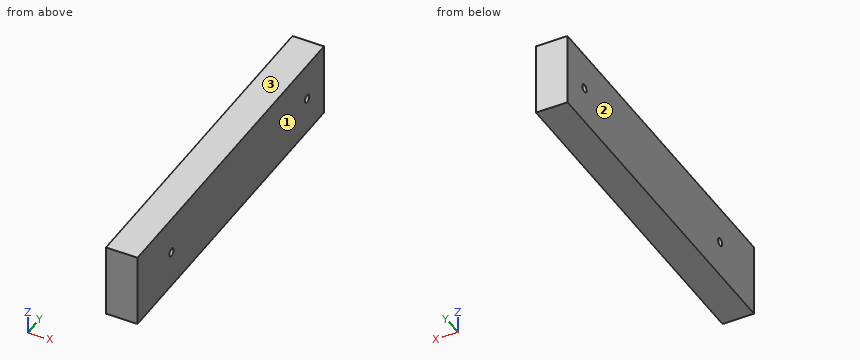
```python
from build123d import *

# Parameters (mm, degrees)
SKETCH1_W           = 38.1
SKETCH1_H           = 88.9
BOSS_EXTRUDE1_DEPTH = 419.1
SKETCH2_OUTSIDE_W   = 176.924
SKETCH2_OUTSIDE_H   = 507.124
SKETCH2_OUTSIDE_W_2 = 88.9
SKETCH2_OUTSIDE_H_2 = 419.1
SKETCH2_OUTSIDE_R   = 4.7625
CUT_EXTRUDE1_DEPTH  = 38.1


with BuildPart() as part:
    # Sketch1 → Boss-Extrude1 (new body)
    with BuildSketch(Plane(origin=(0, 0, 0), x_dir=(1, 0, 0), z_dir=(0, 1, 0))):
        with Locations((19.05, 44.45)):
            Rectangle(SKETCH1_W, SKETCH1_H)
    extrude(amount=BOSS_EXTRUDE1_DEPTH)

    # Sketch2 outside → Cut-Extrude1 (cut)
    # profile 1 of 3: a face of its own
    with BuildSketch(Plane.ZY):
        with Locations((-44.45, 209.55)):
            Rectangle(SKETCH2_OUTSIDE_W, SKETCH2_OUTSIDE_H)
        with Locations((-44.45, 209.55)):
            Rectangle(SKETCH2_OUTSIDE_W_2, SKETCH2_OUTSIDE_H_2, mode=Mode.SUBTRACT)
    # profile 2 of 3: a face of its own
    with BuildSketch(Plane.ZY):
        with Locations((-44.45, 381)):
            Circle(SKETCH2_OUTSIDE_R)
    # profile 3 of 3: a face of its own
    with BuildSketch(Plane.ZY):
        with Locations((-44.45, 76.2)):
            Circle(SKETCH2_OUTSIDE_R)
    extrude(amount=-CUT_EXTRUDE1_DEPTH, mode=Mode.SUBTRACT)


solid = part.part
```
Could you check a few things on this model? Use its own coordinates, in mm. Face numbers are marked on the shaded views. Round coordinates to 2 decimals unless told otherwise and drop trailing zeros. Loops run counter-clockwise (first coordinate to the right, second up) from the corner with the lowest first, then second, coordinate; pieces in that order, holes last. Notation, with made-up numbers: (3.5, 78.5) -> (45.5, 78.5) arc R21 cw to (45.5, 103.5) -> close; hole circle Ø5 at (10.5, -32). An arc over 180 degrees is marked (long way). Put each result on its own line as item: value.
Q1. Thinking about a two-plate mould opening in X: for the marked faces 1, 2 and 3, which applies, pulls with the +X half, pulls with the -X half, needs draft (parallel to the pull), parting line crosses it, or undercut?
Checks:
face 1: pulls with the +X half
face 2: pulls with the -X half
face 3: needs draft
Q2. I want a section at B-B on z = -44.45. Write out the boundary of the cut face in (x, y).
Checks:
outline: (0, 0) -> (38.1, 0) -> (38.1, 71.44) -> (0, 71.44) -> close; (0, 80.96) -> (38.1, 80.96) -> (38.1, 376.24) -> (0, 376.24) -> close; (0, 385.76) -> (38.1, 385.76) -> (38.1, 419.1) -> (0, 419.1) -> close
Q3. Please list where these lines run through material, in increasing order: line 1 (Y direction, x = 28.5, z = -44.45); line 2 (Y direction, x = 17, z = -44); line 3 (Z direction, x = 9, y = 76). Write a range as from..to.
Checks:
line 1: 0..71.44, 80.96..376.24, 385.76..419.1
line 2: 0..71.46, 80.94..376.26, 385.74..419.1
line 3: -88.9..-49.21, -39.69..0
Q4. I want a section at A-A on y = 381. Write out the boundary of the cut face in (x, z).
Checks:
outline: (0, -88.9) -> (38.1, -88.9) -> (38.1, -49.21) -> (0, -49.21) -> close; (0, -39.69) -> (38.1, -39.69) -> (38.1, 0) -> (0, 0) -> close
Q5. For pin 1 Ø10 at (x, y) = (15.5, 340) entering from +Z, with a flat end and sliding along its axis, tell me the tip position at first contact or that it passes through.
Checks:
pin 1: z = 0
